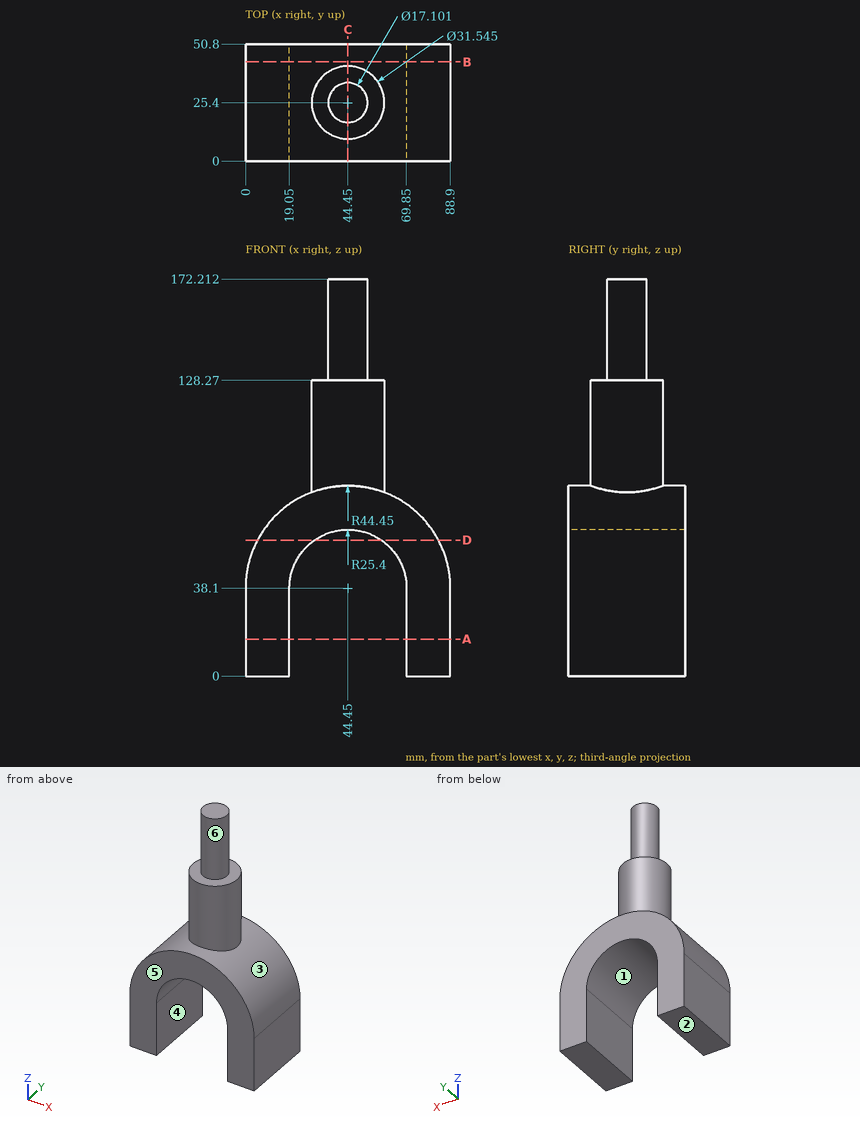
Geometry: see drawing. Coordinates: mm, zero at the bounding-box minimum. A direction names the side the tool comes from. Give positions to 0.01 mm unless a question says otherwise; leave off trailing zeros. Loops run counter-clockwise (first coordinate to the right, second up) from the corner with the lowest first, then second, coordinate; pieces in that order, holes last. Notation, with made-up numbers: M 65.5,21 L 108.5,21 A24 ccw 108.5,50 Z; hole C 27,26 d1. An arc over 180 degrees is marked long. Answer as CSV lines item,"result". Start each with the question number.
1. Section A-A on z = 16. Return loops of the section in (x, y).
2. Section C-C on x = 44.45. Return loops of the section in (y, z).
3. Section D-D on z = 59. Return loops of the section in (x, y) (1 decimal), plus the area to 3 significant figures.
4. Reachability of the marked faces 4, 5 and 6 from +Z, -Z, +X, -X, +Y, -Y: full face, straight path, thin tool, end or side. Return the list, or none.
5. Line query: L1, parallel to X at y = 25, z = 22; L2, parallel to X at y = 34, z = 40; L3, parallel to X at y = 33.5, z = 110 (1 decimal). Output: solid intervals per line, ascending.
6. Pin query (flat end, axial travel): P1, Ø8, axis at x = 45, z = 107, coming from the -Y side; P2, Ø1.5, axis at x = 64, y = 39, coming from the -Z side (1 decimal); P3, Ø1, axis at x = 43, y = 11, coming from the -Z side (1 decimal). Return the tip coordinate at first contact, or that it passes through.
7. Section B-B on y = 43. Return loops of the section in (x, z).
8. Pull-direction query (X, two-part tool) for the marked faces 1, 2 and 3; classes: released by +X, released by -X, zero draft, split by the parting line, or undercut.
Computed values:
1,outline,"M 0,0 L 19.05,0 L 19.05,50.8 L 0,50.8 Z; M 69.85,0 L 88.9,0 L 88.9,50.8 L 69.85,50.8 Z"
2,outline,"M 0,63.5 L 50.8,63.5 L 50.8,82.55 L 41.17,82.55 L 41.17,128.27 L 33.95,128.27 L 33.95,172.21 L 16.85,172.21 L 16.85,128.27 L 9.63,128.27 L 9.63,82.55 L 0,82.55 Z"
3,outline,"M 5.2,0 L 30,0 L 30,50.8 L 5.2,50.8 Z; M 58.9,0 L 83.7,0 L 83.7,50.8 L 58.9,50.8 Z"
3,area,"2,520 mm²"
4,face 4,"-Z, +Y, -Y"
4,face 5,"+Z, -Z, +X, -X, -Y"
4,face 6,"+Z"
5,L1,"x = 0 to 19.05, 69.85 to 88.9"
5,L2,"x = 0.04 to 19.12, 69.78 to 88.86"
5,L3,"x = 30.9 to 58"
6,P1,"stops at y = 9.63"
6,P2,"stops at z = 53.4"
6,P3,"stops at z = 63.4"
7,outline,"M 0,0 L 19.05,0 L 19.05,38.1 A25.4 cw 69.85,38.1 L 69.85,0 L 88.9,0 L 88.9,38.1 A44.45 ccw 0,38.1 Z"
8,face 1,"undercut"
8,face 2,"zero draft"
8,face 3,"split by the parting line"
